Geometry check sheet. Reference: the model listing, model coordinates, mm. A direction names the side the tool comes from. Give positions to 0.01 mm unless a question says otherwise; leave off trailing zeros. Write each loop counter-clockwise with the first axis right and the second up, starting at its lowest first coordinate (ties: lowest second). Pieces come first, ordered by that corner, then holes. Notation, with made-up numbers: (45, -20) -> (63, -20) arc R21 ccw to (63, -7) -> close; hole circle Ø10 at (-35.75, 70.25). An arc over 180 degrees is marked (long way). Write item = value, one per line. Start each with the question number.
1. Cross-section at A-A, the plane x = 480. Record the cut outline in (y, z) (3 decimals), plus the area to 3 significant figures.
2. Depth check by flat-ended pin: P1, Ø3.5, axis at x = 480, y = 93.5, coming from the +Z side; P2, Ø0.9, axis at x = 479.5, z = 105.5, coming from the -Y side; P3, Ø4, axis at x = 486, z = 122.5, coming from the +Y side; P4, Ø5.5, axis at y = 95.5, z = 127, coming from the +X side. Enter the tip coordinate at first touch or a pass-through.
3. Set-up check for faces 1 (the flat face through (479, 92, 125)), 2 (the flat face through (479, 99, 125)), 3 (the flat face through (485.7, 98, 115)), 4 (the cylindrical face through (479.48, 97.01, 127.35)): record each of +Z, -Z, +X, -X, +Y, -Y from which the full face is reachable in a straight line by a thin tool's end or side.
4. Cross-section at C-C, the plane y = 94.5. Record the cut outline in (x, z) (3 decimals).
5. Cross-section at B-B, the plane z = 105. Record the cut outline in (x, y).
6. Thickness scan on line 1 along Z through (x, y) = (482.5, 99.25); line 2 along Y through (x, z) = (479.4, 105); line 3 along Z through (x, y) = (479.85, 95). Record the ranges inside material, lowest first.
7. Mould release check, pull along Z, two halves, no side actions. Record for faces 5 (the flat face through (481, 98, 108.55)), 6 (the flat face through (485.5, 103.3, 119.4)), 7 (the flat face through (486, 90, 115)), 8 (the cylindrical face through (483.6, 95, 107.3)): pulls with the +Z half, pulls with the -Z half, needs draft (parallel to the pull), parting line crosses it, or undercut.
```python
from build123d import *

# Parameters (mm, degrees)
BOX520_W                  = 10.4
BOX520_H                  = 12.4
BOX520_DEPTH              = 27
FILLET403_R               = 1
CYLINDER1231_R            = 8
CYLINDER1231_DEPTH        = 27
CYLINDER1233_R            = 6.5
CYLINDER1233_DEPTH        = 17
CYLINDER1232_R            = 8
CYLINDER1232_DEPTH        = 17
CYLINDER1234_R            = 8
CYLINDER1234_DEPTH        = 27
CUT014272_PLACEMENT_ANGLE = 90
CYLINDER1230_R            = 5.5
CYLINDER1230_DEPTH        = 15
CYLINDER1229_R            = 1.2
CYLINDER1229_DEPTH        = 11
CYLINDER1228_R            = 1.2
CYLINDER1228_DEPTH        = 11
CYLINDER1275_R            = 2.3
CYLINDER1275_DEPTH        = 11
BOX519_W                  = 9.5
BOX519_H                  = 18
BOX519_DEPTH              = 16
CHAMFER036_SIZE2          = 6.5
CHAMFER036_SIZE           = 13
FILLET409_R               = 2.5
BOX542_W                  = 3
BOX542_H                  = 7
BOX542_DEPTH              = 28
FILLET415_R               = 2


with BuildPart() as fillet403:
    # Box520 → Box520 (new body)
    with BuildSketch(Plane(origin=(-5.2, -6.2, 0), x_dir=(1, 0, 0), z_dir=(0, 0, 1))):
        with Locations((5.2, 6.2)):
            Rectangle(BOX520_W, BOX520_H)
    extrude(amount=BOX520_DEPTH)

    # Fillet403
    fillet403_edges = [fillet403.edges().sort_by_distance(p)[0] for p in [
        (-5.2, -6.2, 13.5),
        (-5.2, 6.2, 13.5),
        (5.2, -6.2, 13.5),
        (5.2, 6.2, 13.5),
    ]]
    fillet(fillet403_edges, radius=FILLET403_R)


with BuildPart() as cut014271:
    # Cylinder1231 → Cylinder1231 (new body)
    with BuildSketch(Plane.XY):
        Circle(CYLINDER1231_R)
    extrude(amount=CYLINDER1231_DEPTH)

    # Cut014271: cut Fillet403
    add(fillet403.part, mode=Mode.SUBTRACT)


with BuildPart() as cylinder1429:
    # Cylinder1233 → Cylinder1233 (new body)
    with BuildSketch(Plane.XY):
        Circle(CYLINDER1233_R)
    extrude(amount=CYLINDER1233_DEPTH)


with BuildPart() as fusion248002050137:
    # Cylinder1232 → Cylinder1232 (new body)
    with BuildSketch(Plane.XY):
        Circle(CYLINDER1232_R)
    extrude(amount=CYLINDER1232_DEPTH)

    # Cut014270: cut Cylinder1429
    add(cylinder1429.part, mode=Mode.SUBTRACT)

    # Fusion248002050137: union Cut014271
    add(cut014271.part)


with BuildPart() as bucket_turning_motor002:
    # Cylinder1234 → Cylinder1234 (new body)
    with BuildSketch(Plane.XY):
        Circle(CYLINDER1234_R)
    extrude(amount=CYLINDER1234_DEPTH)

    # Cut014272: cut Fusion248002050137
    add(fusion248002050137.part, mode=Mode.SUBTRACT)


with BuildPart() as bucket_turning_motor002_1:
    # Cut014272 placement: moved
    add(bucket_turning_motor002.part.moved(Location((480.5, 119, 114.75))).rotate(Axis((480.5, 119, 114.75), (1, 0, 0)), CUT014272_PLACEMENT_ANGLE))


with BuildPart() as cylinder1230:
    # Cylinder1230 → Cylinder1230 (new body)
    with BuildSketch(Plane(origin=(480, 92, 115), x_dir=(1, 0, 0), z_dir=(0, -1, 0))):
        Circle(CYLINDER1230_R)
    extrude(amount=CYLINDER1230_DEPTH)


with BuildPart() as cylinder1229:
    # Cylinder1229 → Cylinder1229 (new body)
    with BuildSketch(Plane(origin=(476, 95, 105), x_dir=(0, 0, -1), z_dir=(1, 0, 0))):
        Circle(CYLINDER1229_R)
    extrude(amount=CYLINDER1229_DEPTH)


with BuildPart() as fusion248002050197:
    # Cylinder1228 → Cylinder1228 (new body)
    with BuildSketch(Plane(origin=(476, 96, 128), x_dir=(0, 0, -1), z_dir=(1, 0, 0))):
        Circle(CYLINDER1228_R)
    extrude(amount=CYLINDER1228_DEPTH)

    # Fusion248002050197: union Cylinder1229
    add(cylinder1229.part)


with BuildPart() as cylinder1275:
    # Cylinder1275 → Cylinder1275 (new body)
    with BuildSketch(Plane(origin=(481, 95, 105), x_dir=(0, 0, -1), z_dir=(1, 0, 0))):
        Circle(CYLINDER1275_R)
    extrude(amount=CYLINDER1275_DEPTH)


with BuildPart() as fillet409:
    # Box519 → Box519 (new body)
    with BuildSketch(Plane(origin=(478, 90, 107), x_dir=(1, 0, 0), z_dir=(0, 0, 1))):
        with Locations((4.75, 9)):
            Rectangle(BOX519_W, BOX519_H)
    extrude(amount=BOX519_DEPTH)

    # Chamfer036
    chamfer036_edges = [fillet409.edges().sort_by_distance(p)[0] for p in [
        (482.75, 108, 123),
    ]]
    chamfer036_side = fillet409.faces().sort_by_distance((482.75, 108, 115))[0]
    chamfer(chamfer036_edges, length=CHAMFER036_SIZE, length2=CHAMFER036_SIZE2, reference=chamfer036_side)

    # Fillet409
    fillet409_edges = [fillet409.edges().sort_by_distance(p)[0] for p in [
        (487.5, 95.75, 123),
        (487.5, 99, 107),
    ]]
    fillet(fillet409_edges, radius=FILLET409_R)


with BuildPart() as bucket_rotating_motor_holder:
    # Box542 → Box542 (new body)
    with BuildSketch(Plane(origin=(478, 92, 102), x_dir=(1, 0, 0), z_dir=(0, 0, 1))):
        with Locations((1.5, 3.5)):
            Rectangle(BOX542_W, BOX542_H)
    extrude(amount=BOX542_DEPTH)

    # Fusion248002050208: union Fillet409
    add(fillet409.part)

    # Cut014334: cut Cylinder1275
    add(cylinder1275.part, mode=Mode.SUBTRACT)

    # Cut014335: cut Fusion248002050197
    add(fusion248002050197.part, mode=Mode.SUBTRACT)

    # Cut014336: cut Cylinder1230
    add(cylinder1230.part, mode=Mode.SUBTRACT)

    # Cut014337: cut bucket-turning-motor002
    add(bucket_turning_motor002_1.part, mode=Mode.SUBTRACT)

    # Fillet415
    fillet415_edges = [bucket_rotating_motor_holder.edges().sort_by_distance(p)[0] for p in [
        (479.5, 99, 102),
        (479.5, 92, 102),
        (479.5, 99, 130),
        (479.5, 92, 130),
    ]]
    fillet(fillet415_edges, radius=FILLET415_R)


solid = bucket_rotating_motor_holder.part
```
Answers:
q1.outline = (90, 107) -> (92, 107) -> (92, 104) arc R2 ccw to (94, 102) -> (97, 102) arc R2 ccw to (99, 104) -> (99, 107) -> (108, 107) -> (108, 108.55) -> (92, 108.55) -> (92, 109.5) -> (90, 109.5) -> close; (90, 120.5) -> (92, 120.5) -> (92, 120.95) -> (102.525, 120.95) -> (101.5, 123) -> (99, 123) -> (99, 128) arc R2 ccw to (97, 130) -> (94, 130) arc R2 ccw to (92, 128) -> (92, 123) -> (90, 123) -> close; hole circle Ø2.4 at (95, 105); hole circle Ø2.4 at (96, 128)
q1.area = 127 mm^2
q2.P1 = 130
q2.P2 = 92
q2.P3 = 102.75
q2.P4 = 481
q3.face_1 = +Z, +X, -X, -Y
q3.face_2 = +Z, +X, -X, +Y
q3.face_3 = -X
q3.face_4 = +X, -X
q4.outline = (478, 102) -> (481, 102) -> (481, 103.909) -> (478, 103.909) -> close; (478, 106.091) -> (481, 106.091) -> (481, 107.245) -> (486.079, 107.245) arc R2.5 ccw to (487.5, 109.5) -> (487.5, 120.5) arc R2.5 ccw to (485, 123) -> (481, 123) -> (481, 130) -> (478, 130) -> (478, 120.95) -> (484.7, 120.95) arc R1 cw to (485.7, 119.95) -> (485.7, 109.55) arc R1 cw to (484.7, 108.55) -> (478, 108.55) -> close
q5.outline = (478, 92) -> (481, 92) -> (481, 93.8) -> (478, 93.8) -> close; (478, 96.2) -> (481, 96.2) -> (481, 99) -> (478, 99) -> close
q6.line_1 = 107 to 108.55, 120.95 to 123
q6.line_2 = 92 to 93.8, 96.2 to 99
q6.line_3 = 102 to 103.8, 106.2 to 108.55, 120.95 to 127.34, 128.66 to 130
q7.face_5 = undercut
q7.face_6 = pulls with the +Z half
q7.face_7 = needs draft
q7.face_8 = pulls with the -Z half
